```python
from build123d import *

# Parameters (mm, degrees)
SKETCH1_W           = 94
SKETCH1_H           = 84
BOSS_EXTRUDE1_DEPTH = 27
SKETCH2_W           = 90
SKETCH2_H           = 80
CUT_EXTRUDE1_DEPTH  = 25
FILLET2_R           = 5
FILLET3_R           = 5
SKETCH3_R           = 2
BOSS_EXTRUDE2_DEPTH = 10
SKETCH4_R           = 1.6
BOSS_EXTRUDE3_DEPTH = 10
SKETCH5_R           = 1.6
CUT_EXTRUDE2_DEPTH  = 10
SKETCH6_R           = 2
BOSS_EXTRUDE4_DEPTH = 10
SKETCH12_W          = 67
SKETCH12_H          = 37
BOSS_EXTRUDE5_DEPTH = 18
SKETCH13_W          = 65
SKETCH13_H          = 36
CUT_EXTRUDE4_DEPTH  = 18
SKETCH14_W          = 17
SKETCH14_H          = 4
CUT_EXTRUDE5_DEPTH  = 1
SKETCH16_W          = 7
SKETCH16_H          = 3
CUT_EXTRUDE6_DEPTH  = 1
SKETCH17_R          = 2
BOSS_EXTRUDE6_DEPTH = 5
SKETCH18_R          = 1.6
CUT_EXTRUDE7_DEPTH  = 2
CUT_EXTRUDE8_START  = -2
SKETCH19_R          = 1.6
CUT_EXTRUDE8_DEPTH  = 2


with BuildPart() as part:
    # Sketch1 → Boss-Extrude1 (new body)
    with BuildSketch(Plane(origin=(0, 0, 0), x_dir=(1, 0, 0), z_dir=(0, 1, 0))):
        Rectangle(SKETCH1_W, SKETCH1_H)
    extrude(amount=BOSS_EXTRUDE1_DEPTH)

    # Sketch2 → Cut-Extrude1 (cut)
    with BuildSketch(Plane(origin=(0, 27, 0), x_dir=(1, 0, 0), z_dir=(0, 1, 0))):
        Rectangle(SKETCH2_W, SKETCH2_H)
    extrude(amount=-CUT_EXTRUDE1_DEPTH, mode=Mode.SUBTRACT)

    # Fillet2
    fillet2_edges = [part.edges().sort_by_distance(p)[0] for p in [
        (0, 0, 42),
        (-47, 0, 0),
        (0, 0, -42),
        (47, 0, 0),
        (47, 13.5, 42),
        (-47, 13.5, 42),
        (-47, 13.5, -42),
        (47, 13.5, -42),
    ]]
    fillet(fillet2_edges, radius=FILLET2_R)

    # Fillet3
    fillet3_edges = [part.edges().sort_by_distance(p)[0] for p in [
        (45, 14.5, -40),
        (45, 14.5, 40),
        (-45, 14.5, 40),
        (-45, 14.5, -40),
    ]]
    fillet(fillet3_edges, radius=FILLET3_R)

    # Sketch3 → Boss-Extrude2 (add)
    with BuildSketch(Plane(origin=(0, 2, 0), x_dir=(1, 0, 0), z_dir=(0, 1, 0))):
        with Locations(Location((33.5, -35, 0), (0, 0, 270))):
            Circle(SKETCH3_R)
        with Locations(Location((33.5, -4, 0), (0, 0, 270))):
            Circle(SKETCH3_R)
        with Locations(Location((-17.5, -4, 0), (0, 0, 270))):
            Circle(SKETCH3_R)
        with Locations(Location((-17.5, -35, 0), (0, 0, 270))):
            Circle(SKETCH3_R)
    extrude(amount=BOSS_EXTRUDE2_DEPTH)

    # Sketch4 → Boss-Extrude3 (add)
    with BuildSketch(Plane(origin=(0, 12, 0), x_dir=(1, 0, 0), z_dir=(0, 1, 0))):
        with Locations((-17.5, -4)):
            Circle(SKETCH4_R)
        with Locations((33.5, -4)):
            Circle(SKETCH4_R)
        with Locations((-17.5, -35)):
            Circle(SKETCH4_R)
        with Locations((33.5, -35)):
            Circle(SKETCH4_R)
    extrude(amount=-BOSS_EXTRUDE3_DEPTH)

    # Sketch5 → Cut-Extrude2 (cut)
    with BuildSketch(Plane(origin=(0, 12, 0), x_dir=(1, 0, 0), z_dir=(0, 1, 0))):
        with Locations(Location((-17.5, -4, 0), (0, 0, 270))):
            Circle(SKETCH5_R)
        with Locations(Location((33.5, -4, 0), (0, 0, 270))):
            Circle(SKETCH5_R)
        with Locations(Location((-17.5, -35, 0), (0, 0, 270))):
            Circle(SKETCH5_R)
        with Locations(Location((33.5, -35, 0), (0, 0, 270))):
            Circle(SKETCH5_R)
    extrude(amount=-CUT_EXTRUDE2_DEPTH, mode=Mode.SUBTRACT)

    # Sketch6 → Boss-Extrude4 (add)
    with BuildSketch(Plane(origin=(0, 2, 0), x_dir=(1, 0, 0), z_dir=(0, 1, 0))):
        with Locations(Location((-33, -35, 0), (0, 0, 270))):
            Circle(SKETCH6_R)
        with Locations(Location((-33, -17, 0), (0, 0, 270))):
            Circle(SKETCH6_R)
    extrude(amount=BOSS_EXTRUDE4_DEPTH)

    # Sketch12 → Boss-Extrude5 (add)
    with BuildSketch(Plane(origin=(0, 2, 0), x_dir=(1, 0, 0), z_dir=(0, 1, 0))):
        with Locations((7.45155259, 21.5)):
            Rectangle(SKETCH12_W, SKETCH12_H)
    extrude(amount=BOSS_EXTRUDE5_DEPTH)

    # Sketch13 → Cut-Extrude4 (cut)
    with BuildSketch(Plane(origin=(0, 20, 0), x_dir=(1, 0, 0), z_dir=(0, 1, 0))):
        with Locations((7.45155259, 22)):
            Rectangle(SKETCH13_W, SKETCH13_H)
    extrude(amount=-CUT_EXTRUDE4_DEPTH, mode=Mode.SUBTRACT)

    # Sketch14 → Cut-Extrude5 (cut)
    with BuildSketch(Plane(origin=(0, 0, 40), x_dir=(-1, 0, 0), z_dir=(0, 0, -1))):
        with Locations((31.5, 14)):
            Rectangle(SKETCH14_W, SKETCH14_H)
    extrude(amount=-CUT_EXTRUDE5_DEPTH, mode=Mode.SUBTRACT)

    # Sketch16 → Cut-Extrude6 (cut)
    with BuildSketch(Plane(origin=(0, 0, 41), x_dir=(-1, 0, 0), z_dir=(0, 0, -1))):
        with Locations((31.5, 14.5)):
            Rectangle(SKETCH16_W, SKETCH16_H)
    extrude(amount=-CUT_EXTRUDE6_DEPTH, mode=Mode.SUBTRACT)

    # Sketch17 → Boss-Extrude6 (add)
    with BuildSketch(Plane(origin=(-45, 0, 0), x_dir=(0, 0, -1), z_dir=(1, 0, 0))):
        with Locations(Location((25, 7, 0), (0, 0, 180))):
            Circle(SKETCH17_R)
        with Locations(Location((5, 7, 0), (0, 0, 180))):
            Circle(SKETCH17_R)
    extrude(amount=BOSS_EXTRUDE6_DEPTH)

    # Sketch18 → Cut-Extrude7 (cut)
    with BuildSketch(Plane(origin=(-45, 0, 0), x_dir=(0, 0, -1), z_dir=(1, 0, 0))):
        with Locations((29, 24.5)):
            Circle(SKETCH18_R)
        with Locations((-29, 24.5)):
            Circle(SKETCH18_R)
    extrude(amount=-CUT_EXTRUDE7_DEPTH, mode=Mode.SUBTRACT)

    # Sketch19 → Cut-Extrude8 (cut)
    with BuildSketch(Plane.ZY.offset(-45).offset(CUT_EXTRUDE8_START)):
        with Locations(Location((-29, 24.5, 0), (0, 0, 180))):
            Circle(SKETCH19_R)
        with Locations(Location((29, 24.5, 0), (0, 0, 180))):
            Circle(SKETCH19_R)
    extrude(amount=CUT_EXTRUDE8_DEPTH, mode=Mode.SUBTRACT)


solid = part.part
```
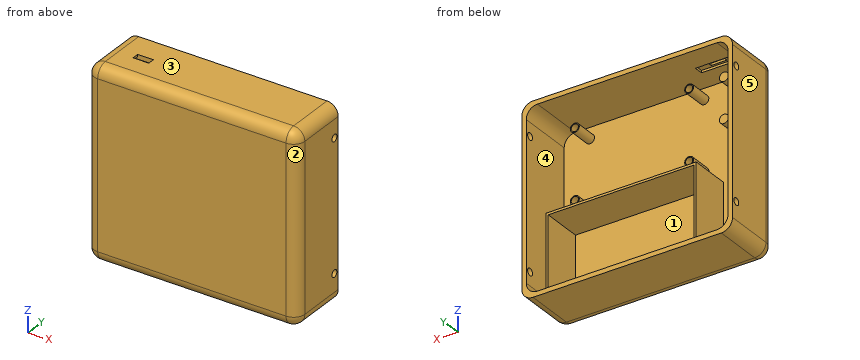
Can you work these out from the model? Positions are in its coordinate system, mm. Face numbers are marked on the shaded views. A direction names the side the tool comes from. Coordinates: 2 decimals unless noted, no trailing zeros. Write each loop counter-clockwise with the first axis right and the second up, starting at its lowest first coordinate (ties: lowest second). Pieces come first, ordered by that corner, then holes. Notation, with made-up numbers: M 60,45.25 L 85,45.25 A23 ccw 85,63.25 Z; hole C 18.5,-29.75 d9. An arc over 180 degrees is marked long. Write item = value, one per line. Start each with the question number.
Q1. On a 3-axis mill with a long thin cutter (end or side, diameter ignored), from which of +Z, -Z, +X, -X, +Y, -Y can I reach the whole of each face in a straight line? I mean the marked faces 1 and 2. Say none if no direction works.
Q2. If we section it at C-C, the plane z = 29: Write out the boundary of the cut face in (x, y).
Q3. If I drill on L1, parallel to X at y = 13, z = -5; L2, parallel to Z at x = -18.5, y = 16.75; L3, parallel to X at y = 18.25, z = 7, over which ranges is the centre line in solid material (lowest first)? Write a range as [from, to].
Q4. If we section it at A-A, the plane x = -33: Write out the boundary of the cut face in (y, z), then the cut area to 3 significant figures.
Q5. Thinking about a two-plate mould opening in X: for the marked faces 3, 4 and 5, which applies, released by +X, released by -X, zero draft, split by the parting line, or undercut?
Q6. If we section it at B-B, the plane y = 21.25: Write out the boundary of the cut face in (x, z).
Q7. I'm going to push flat-ended pins straight in: pin 1 (12 mm diameter, centred on x = 7.5, z = 23, fed in from +Y); pin 2 (5 mm diameter, centred on x = -17.5, z = 35, fed in from +Y); pin 3 (0.5 mm diameter, centred on y = 15, z = 41.5, fed in from -X). Where does each tip first touch, or does it pass through?
Q8. If we section it at D-D, the plane z = 9: Write out the boundary of the cut face in (x, y), then the cut area to 3 significant figures.
Check sheet entries:
q1.face_1 = +Y
q1.face_2 = +Z, -Z, +X, -Y
q2.outline = M -47,5 A5 ccw -42,0 L 42,0 A5 ccw 47,5 L 47,22.9 L 45,22.9 L 45,2 L -45,2 L -45,22.9 L -47,22.9 Z; M -47,26.1 L -45,26.1 L -45,27 L -47,27 Z; M 45,26.1 L 47,26.1 L 47,27 L 45,27 Z
q3.L1 = [-47, -45], [-26.05, -25.05], [39.95, 40.95], [45, 47]
q3.L2 = [-42, -40], [-4, -3], [40, 42]
q3.L3 = [-47, -45], [45, 47]
q4.outline = M 0,-37 A5 ccw 5,-42 L 27,-42 L 27,-40 L 2,-40 L 2,15 L 12,15 L 12,19 L 2,19 L 2,33 L 12,33 L 12,37 L 2,37 L 2,40 L 12,40 L 12,41 L 13,41 L 13,42 L 5,42 A5 ccw 0,37 Z; M 16,40 L 27,40 L 27,42 L 16,42 Z
q4.area = 330 mm²
q5.face_3 = zero draft
q5.face_4 = undercut
q5.face_5 = released by -X
q6.outline = M -47,-37 A5 ccw -42,-42 L 42,-42 A5 ccw 47,-37 L 47,37 A5 ccw 42,42 L -42,42 A5 ccw -47,37 Z; hole M -45,-35 A5 ccw -40,-40 L 40,-40 A5 ccw 45,-35 L 45,35 A5 ccw 40,40 L -40,40 A5 ccw -45,35 Z
q7.pin_1 = 2
q7.pin_2 = 12
q7.pin_3 = -44.63
q8.outline = M -47,5 A5 ccw -42,0 L 42,0 A5 ccw 47,5 L 47,27 L 45,27 L 45,2 L -45,2 L -45,27 L -47,27 Z
q8.area = 277 mm²
